For this review, take the finished solid that the model builds, in its own axes (mm). Coordinates: 2 decimals unless noted, no trailing zeros. Write each loop counter-clockwise with the first axis right and the second up, starting at its lowest first coordinate (ties: lowest second). Pieces come first, ordered by that corner, then holes. Notation, with made-up numbers: (1.25, 64) - (9.25, 64) arc R25 ccw to (9.25, 97) - close; hole circle Ø11 at (0, 83). An arc over 180 degrees is marked (long way). Use one line per item in the form item = value. Start each with the question number.
1) We need section D-D (x = -109.5). Give the boundary of the cut face in (y, z).
2) We need section B-B (z = 0.55). Give the boundary of the cut face in (x, y), plus the area to 3 significant figures.
3) For L1, parallel to Y at x = -108, z = 0.95; L2, parallel to Y at x = -109.5, z = 1.4; L3, parallel to X at y = 66, z = 0.5, list the stretches that pass through material, from the lowest coordinate up. Write a range as from..to.
4) We need section C-C (y = 56). Give the boundary of the cut face in (x, z), plus the area to 3 significant figures.
5) Insertion check: P1, Ø2, axis at x = -105, y = 50, coming from the +Z side. The pin has a flat end and moves straight along its axis. Give the tip position at first contact, or say it passes through.
6) We need section A-A (x = -103). Give the boundary of the cut face in (y, z).
7) Mouldability with a two-part tool opening along X and no side actions: class faces 1 (the cylindrical face through (-114.17, 34.35, 0.78)), 2 (the flat face through (-100.593, 52, 1)), 3 (the cylindrical face through (-105.325, 46.241, 0.805)) as pulls with the +X half, pulls with the -X half, needs draft (parallel to the pull), parting line crosses it, or undercut.
```python
from build123d import *

# Parameters (mm, degrees)
SKETCH1_W           = 101.6
SKETCH1_H           = 101.6
BOSS_EXTRUDE1_DEPTH = 1.5875
SKETCH2_R           = 5.999999938
CUT_EXTRUDE1_DEPTH  = 190.018384556
SKETCH4_R           = 1.778
CUT_EXTRUDE2_DEPTH  = 190.018384556
SKETCH5_W           = 43.3
SKETCH5_H           = 101.6
CUT_EXTRUDE4_DEPTH  = 190.018384556
SKETCH10_W          = 15
SKETCH10_H          = 31.816690228
SKETCH10_H_2        = 32.081483739
CUT_EXTRUDE5_DEPTH  = 155.410769427
FILLET1_R           = 5


with BuildPart() as part:
    # Sketch1 → Boss-Extrude1 (new body)
    with BuildSketch(Plane.XY):
        with Locations((-108.093233083, 51.563909774)):
            Rectangle(SKETCH1_W, SKETCH1_H)
    extrude(amount=BOSS_EXTRUDE1_DEPTH)

    # Sketch2 → Cut-Extrude1 (cut, through all)
    with BuildSketch(Plane.XY.offset(1.5875)):
        with Locations((-108.093233083, 51.563909774)):
            Circle(SKETCH2_R)
    extrude(amount=-CUT_EXTRUDE1_DEPTH, mode=Mode.SUBTRACT)

    # Sketch4 → Cut-Extrude2 (cut, through all)
    with BuildSketch(Plane.XY.offset(1.5875)):
        with Locations((-108.093233083, 66.360241624)):
            Circle(SKETCH4_R)
        with Locations((-108.093233083, 36.767577924)):
            Circle(SKETCH4_R)
    extrude(amount=-CUT_EXTRUDE2_DEPTH, mode=Mode.SUBTRACT)

    # Sketch5 → Cut-Extrude4 (cut, through all)
    with BuildSketch(Plane.XY.offset(1.5875)):
        with Locations((-137.243233083, 51.563909774)):
            Rectangle(SKETCH5_W, SKETCH5_H)
        with Locations((-78.943233083, 51.563909774)):
            Rectangle(SKETCH5_W, SKETCH5_H)
    extrude(amount=-CUT_EXTRUDE4_DEPTH, mode=Mode.SUBTRACT)

    # Sketch10 → Cut-Extrude5 (cut, through all)
    with BuildSketch(Plane.XY.offset(1.5875)):
        with Locations((-108.093233083, 86.45556466)):
            Rectangle(SKETCH10_W, SKETCH10_H)
        with Locations((-108.093233083, 16.804651644)):
            Rectangle(SKETCH10_W, SKETCH10_H_2)
    extrude(amount=-CUT_EXTRUDE5_DEPTH, mode=Mode.SUBTRACT)

    # Fillet1
    fillet1_edges = [part.edges().sort_by_distance(p)[0] for p in [
        (-115.593233083, 70.547219546, 0.79375),
        (-100.593233083, 70.547219546, 0.79375),
        (-100.593233083, 32.845393513, 0.79375),
        (-115.593233083, 32.845393513, 0.79375),
    ]]
    fillet(fillet1_edges, radius=FILLET1_R)


solid = part.part
```
Determined:
q1.outline = (32.85, 0) - (35.68, 0) - (35.68, 1.59) - (32.85, 1.59) - close; (37.85, 0) - (45.73, 0) - (45.73, 1.59) - (37.85, 1.59) - close; (57.4, 0) - (65.27, 0) - (65.27, 1.59) - (57.4, 1.59) - close; (67.45, 0) - (70.55, 0) - (70.55, 1.59) - (67.45, 1.59) - close
q2.outline = (-115.59, 37.85) arc R5 ccw to (-110.59, 32.85) - (-105.59, 32.85) arc R5 ccw to (-100.59, 37.85) - (-100.59, 65.55) arc R5 ccw to (-105.59, 70.55) - (-110.59, 70.55) arc R5 ccw to (-115.59, 65.55) - close; hole circle Ø12 at (-108.09, 51.56); hole circle Ø3.56 at (-108.09, 36.77); hole circle Ø3.56 at (-108.09, 66.36)
q2.area = 411 mm²
q3.L1 = 32.85..34.99, 38.54..45.56, 57.56..64.58, 68.14..70.55
q3.L2 = 32.85..35.68, 37.85..45.73, 57.4..65.27, 67.45..70.55
q3.L3 = -115.57..-109.83, -106.35..-100.61
q4.outline = (-115.59, 0) - (-112.13, 0) - (-112.13, 1.59) - (-115.59, 1.59) - close; (-104.05, 0) - (-100.59, 0) - (-100.59, 1.59) - (-104.05, 1.59) - close
q4.area = 11.0 mm²
q5.P1 = through
q6.outline = (33.57, 0) - (48.39, 0) - (48.39, 1.59) - (33.57, 1.59) - close; (54.74, 0) - (69.82, 0) - (69.82, 1.59) - (54.74, 1.59) - close
q7.face_1 = pulls with the -X half
q7.face_2 = pulls with the +X half
q7.face_3 = undercut
